Design review of the part built by this model. Coordinates are the model's own, in mm. Round coordinates to 2 decimals unless told otherwise and drop trailing zeros. Order: outer loops, then holes, each group sorted by start corner. A loop starts at its lowest first (then second) coordinate and runs counter-clockwise, first axis right, second up.
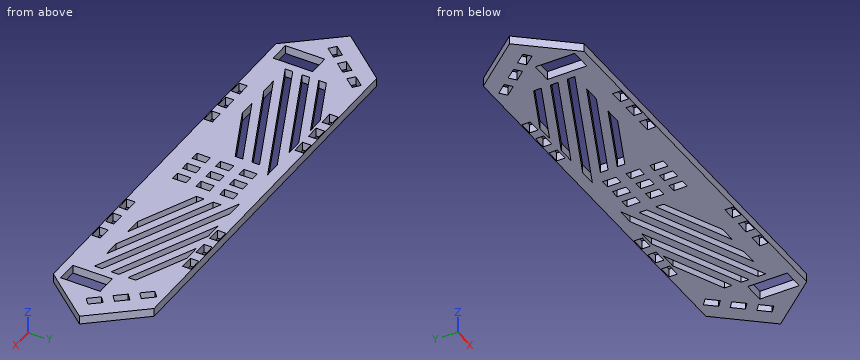
from build123d import *

# Parameters (mm, degrees)
SKETCH_1_W      = 12.5
SKETCH_1_H      = 23.5
SKETCH_1_W_2    = 5
SKETCH_1_H_2    = 8
SKETCH_1_W_3    = 8
SKETCH_1_H_3    = 5
EXTRUDE_1_DEPTH = 5


with BuildPart() as part:
    # 草图1 → 凸台-拉伸1 (new body)
    with BuildSketch(Plane.XY):
        Polygon((140, 0), (115, -30), (-115, -30), (-140, 0), (-115, 30), (115, 30), align=None)
        Polygon((-105.700921998, 26.158893602), (-110.822397196, 20.013123365), (-106.981290798, 16.812201367), (-101.8598156, 22.957971604), align=None, mode=Mode.SUBTRACT)
        Polygon((-114.663503594, 15.403795688), (-119.784978791, 9.258025451), (-115.943872393, 6.057103453), (-110.822397196, 12.202873689), align=None, mode=Mode.SUBTRACT)
        Polygon((-123.626085189, 4.648697773), (-128.747560386, -1.497072463), (-124.906453988, -4.697994462), (-119.784978791, 1.447775775), align=None, mode=Mode.SUBTRACT)
        Polygon((-98.5, -0.47150647), (-46.579460947, 23), (-36.579460947, 23), (-98.5, -4.992165712), (-98.5, -3), align=None, mode=Mode.SUBTRACT)
        with Locations((-109.75, -13.25)):
            Rectangle(SKETCH_1_W, SKETCH_1_H, mode=Mode.SUBTRACT)
        Rectangle(SKETCH_1_W_2, SKETCH_1_H_2, mode=Mode.SUBTRACT)
        with Locations((0, 14)):
            Rectangle(SKETCH_1_W_2, SKETCH_1_H_2, mode=Mode.SUBTRACT)
        with Locations((0, -14)):
            Rectangle(SKETCH_1_W_2, SKETCH_1_H_2, mode=Mode.SUBTRACT)
        Polygon((-98.5, -10.479340758), (-24.441463471, 23), (-14.441463471, 23), (-98.5, -15), align=None, mode=Mode.SUBTRACT)
        Polygon((-20, 15), (-86.362002523, -15), (-76.362002523, -15), (-20, 10.479340758), align=None, mode=Mode.SUBTRACT)
        Polygon((-20, 4.992165712), (-64.224005046, -15), (-54.224005046, -15), (-20, 0.47150647), align=None, mode=Mode.SUBTRACT)
        Polygon((-58.717458424, 23), (-68.717458424, 23), (-98.5, 9.536327819), (-98.5, 5.015668577), align=None, mode=Mode.SUBTRACT)
        Polygon((98.5, 5.015668577), (58.717458424, 23), (68.717458424, 23), (98.5, 9.536327819), align=None, mode=Mode.SUBTRACT)
        Polygon((20, 0.47150647), (20, 4.992165712), (64.224005046, -15), (54.224005046, -15), align=None, mode=Mode.SUBTRACT)
        Polygon((98.5, -15), (98.5, -10.479340758), (24.441463471, 23), (14.441463471, 23), align=None, mode=Mode.SUBTRACT)
        Polygon((20, 10.479340758), (20, 15), (86.362002523, -15), (76.362002523, -15), align=None, mode=Mode.SUBTRACT)
        Polygon((98.5, -0.47150647), (98.5, -3), (98.5, -4.992165712), (36.579460947, 23), (46.579460947, 23), align=None, mode=Mode.SUBTRACT)
        with Locations((109.75, -13.25)):
            Rectangle(SKETCH_1_W, SKETCH_1_H, mode=Mode.SUBTRACT)
        Polygon((119.784978791, 1.447775775), (124.906453988, -4.697994462), (128.747560386, -1.497072463), (123.626085189, 4.648697773), align=None, mode=Mode.SUBTRACT)
        Polygon((110.822397196, 12.202873689), (115.943872393, 6.057103453), (119.784978791, 9.258025451), (114.663503594, 15.403795688), align=None, mode=Mode.SUBTRACT)
        Polygon((101.8598156, 22.957971604), (106.981290798, 16.812201367), (110.822397196, 20.013123365), (105.700921998, 26.158893602), align=None, mode=Mode.SUBTRACT)
        with Locations((-10, 0)):
            Rectangle(SKETCH_1_W_2, SKETCH_1_H_2, mode=Mode.SUBTRACT)
        with Locations((-10, 14)):
            Rectangle(SKETCH_1_W_2, SKETCH_1_H_2, mode=Mode.SUBTRACT)
        with Locations((-10, -14)):
            Rectangle(SKETCH_1_W_2, SKETCH_1_H_2, mode=Mode.SUBTRACT)
        with Locations((10, -14)):
            Rectangle(SKETCH_1_W_2, SKETCH_1_H_2, mode=Mode.SUBTRACT)
        with Locations((10, 14)):
            Rectangle(SKETCH_1_W_2, SKETCH_1_H_2, mode=Mode.SUBTRACT)
        with Locations((10, 0)):
            Rectangle(SKETCH_1_W_2, SKETCH_1_H_2, mode=Mode.SUBTRACT)
        with Locations((-58, 27)):
            Rectangle(SKETCH_1_W_3, SKETCH_1_H_3, mode=Mode.SUBTRACT)
        with Locations((-72, 27)):
            Rectangle(SKETCH_1_W_3, SKETCH_1_H_3, mode=Mode.SUBTRACT)
        with Locations((-44, 27)):
            Rectangle(SKETCH_1_W_3, SKETCH_1_H_3, mode=Mode.SUBTRACT)
        with Locations((58, -27)):
            Rectangle(SKETCH_1_W_3, SKETCH_1_H_3, mode=Mode.SUBTRACT)
        with Locations((72, -27)):
            Rectangle(SKETCH_1_W_3, SKETCH_1_H_3, mode=Mode.SUBTRACT)
        with Locations((44, 27)):
            Rectangle(SKETCH_1_W_3, SKETCH_1_H_3, mode=Mode.SUBTRACT)
        with Locations((58, 27)):
            Rectangle(SKETCH_1_W_3, SKETCH_1_H_3, mode=Mode.SUBTRACT)
        with Locations((72, 27)):
            Rectangle(SKETCH_1_W_3, SKETCH_1_H_3, mode=Mode.SUBTRACT)
        with Locations((44, -27)):
            Rectangle(SKETCH_1_W_3, SKETCH_1_H_3, mode=Mode.SUBTRACT)
        with Locations((-44, -27)):
            Rectangle(SKETCH_1_W_3, SKETCH_1_H_3, mode=Mode.SUBTRACT)
        with Locations((-58, -27)):
            Rectangle(SKETCH_1_W_3, SKETCH_1_H_3, mode=Mode.SUBTRACT)
        with Locations((-72, -27)):
            Rectangle(SKETCH_1_W_3, SKETCH_1_H_3, mode=Mode.SUBTRACT)
    extrude(amount=EXTRUDE_1_DEPTH)


solid = part.part
1) Clearance check with flat-ended pins moving along their axes: P1, Ø3, axis at y = 19, z = 3.5, coming from the -X side; P2, Ø8, axis at x = 66.5, y = 5.5, coming from the -Z side; P3, Ø2.5, axis at y = -28, z = 2.5, coming from the +X side; P4, Ø2.5, axis at y = 13.5, z = 2, coming from the +X side. State where each tip first meets the part, or that it passes through.
Results:
P1: stops at x = -125.42
P2: stops at z = 0
P3: stops at x = 117.71
P4: stops at x = 129.79
2) Take a section at B-B on z = 2.2. State how many separate pieces and enclosed holes the cut face has, plus the area to 3 significant figures.
Results:
separate pieces: 1
enclosed holes: 39
area: 11,200 mm2
3) To check wall thickness, follow line 1 along Y through (x, z) = (85.5, 0.4); line 2 along Y through (x, z) = (-37.5, 2.15); line 3 along X through (y, z) = (-22.5, 3.05). State the ranges of each line that lie inside material, in increasing order.
Results:
line 1: y = -30 to -15, -14.61 to -9.12, -4.6 to 0.88, 5.41 to 10.89, 15.41 to 30
line 2: y = -30 to -7.44, -2.92 to 2.57, 7.09 to 12.58, 17.1 to 22.58, 23 to 30
line 3: x = -121.25 to -116, -103.5 to 103.5, 116 to 121.25
4) Take a section at A-A on x = 81. Give the boundary of the cut face in (y, z), plus the area to 3 significant figures.
Results:
outline: (-30, 0) - (-15, 0) - (-15, 5) - (-30, 5) - close; (-12.58, 0) - (-7.09, 0) - (-7.09, 5) - (-12.58, 5) - close; (-2.57, 0) - (2.92, 0) - (2.92, 5) - (-2.57, 5) - close; (7.44, 0) - (12.93, 0) - (12.93, 5) - (7.44, 5) - close; (17.45, 0) - (30, 0) - (30, 5) - (17.45, 5) - close
area: 220 mm2
